Read the model definition and answer for the solid it produces. Units are mm, in the model's axes. A direction names the side the tool comes from. Coordinates: 2 decimals unless noted, no trailing zeros. Loops run counter-clockwise (first coordinate to the right, second up) from the corner with the lowest first, then second, coordinate; pieces in that order, holes last.
from build123d import *

# Parameters (mm, degrees)
SKETCH_1_R          = 1.45
EXTRUDE_1_DEPTH     = 5
EXTRUDE_2_DEPTH     = 5
FILLET_1_R          = 10
FILLET_2_R          = 2.5
CUT_EXTRUDE_1_DEPTH = 183.793945183
FILLET_3_R          = 3


with BuildPart() as part:
    # 草图1 → 凸台-拉伸1 (new body)
    with BuildSketch(Plane.XY):
        Polygon((-7.5, -7.5), (-7.5, 135.890872965), (13.765981284, 135.890872965), (23.715728753, 125.941125497), (5, 107.225396744), (5, 5), (39.953318806, 5), (79.577164466, 44.623845661), (73.213203436, 50.987806691), (85.941125497, 63.715728753), (122.156854249, 27.5), (122.156854249, -7.5), align=None)
        Circle(SKETCH_1_R, mode=Mode.SUBTRACT)
        with Locations((0, 15)):
            Circle(SKETCH_1_R, mode=Mode.SUBTRACT)
        with Locations((0, 35)):
            Circle(SKETCH_1_R, mode=Mode.SUBTRACT)
        with Locations((15, 0)):
            Circle(SKETCH_1_R, mode=Mode.SUBTRACT)
        with Locations((35, 0)):
            Circle(SKETCH_1_R, mode=Mode.SUBTRACT)
        with Locations((18.058874503, 125.941125497)):
            Circle(SKETCH_1_R, mode=Mode.SUBTRACT)
        with Locations((13.109127035, 130.890872965)):
            Circle(SKETCH_1_R, mode=Mode.SUBTRACT)
        with Locations((6.038059223, 123.819805153)):
            Circle(SKETCH_1_R, mode=Mode.SUBTRACT)
        with Locations((10.987806691, 118.870057685)):
            Circle(SKETCH_1_R, mode=Mode.SUBTRACT)
        with Locations((90.890872965, 53.109127035)):
            Circle(SKETCH_1_R, mode=Mode.SUBTRACT)
        with Locations((85.941125497, 58.058874503)):
            Circle(SKETCH_1_R, mode=Mode.SUBTRACT)
        with Locations((78.870057685, 50.987806691)):
            Circle(SKETCH_1_R, mode=Mode.SUBTRACT)
        with Locations((83.819805153, 46.038059223)):
            Circle(SKETCH_1_R, mode=Mode.SUBTRACT)
        with Locations((0, 125)):
            Circle(SKETCH_1_R, mode=Mode.SUBTRACT)
        with Locations((0, 105)):
            Circle(SKETCH_1_R, mode=Mode.SUBTRACT)
        with Locations((70, 0)):
            Circle(SKETCH_1_R, mode=Mode.SUBTRACT)
        with Locations((90, 0)):
            Circle(SKETCH_1_R, mode=Mode.SUBTRACT)
        Polygon((94.567828227, 48.01795821), (51.549870017, 5), (115.156854249, 5), (115.156854249, 27.428932188), align=None, mode=Mode.SUBTRACT)
    extrude(amount=EXTRUDE_1_DEPTH)

    # 草图3 → 凸台-拉伸2 (add)
    with BuildSketch(Plane.XY):
        Polygon((97.567828227, 45.01795821), (97.567828227, 5), (85.567828227, 5), (68.558849122, 22.008979105), (74.215703372, 27.665833355), (87.567828227, 14.313708499), (87.567828227, 41.01795821), (94.567828227, 48.01795821), align=None)
        Polygon((73.213203436, 50.987806691), (5, 29.379876147), (5, 21), (24.533181149, 27.187535555), (31.561537876, 5), (39.953318806, 5), (32.159691009, 29.603388895), (79.577164466, 44.623845661), align=None)
    extrude(amount=EXTRUDE_2_DEPTH)

    # 圆角1
    fillet_1_edges = [part.edges().sort_by_distance(p)[0] for p in [
        (5, 29.379876147, 2.5),
    ]]
    fillet(fillet_1_edges, radius=FILLET_1_R)

    # 圆角2
    fillet_2_edges = [part.edges().sort_by_distance(p)[0] for p in [
        (97.567828227, 5, 2.5),
        (85.567828227, 5, 2.5),
        (68.558849122, 22.008979105, 2.5),
        (74.215703372, 27.665833355, 2.5),
        (87.567828227, 14.313708499, 2.5),
        (87.567828227, 41.01795821, 2.5),
        (97.567828227, 45.01795821, 2.5),
        (32.159691009, 29.603388895, 2.5),
        (31.561537876, 5, 2.5),
        (24.533181149, 27.187535555, 2.5),
        (5, 21, 2.5),
        (5, 5, 2.5),
        (39.953318806, 5, 2.5),
        (79.577164466, 44.623845661, 2.5),
        (115.156854249, 27.428932188, 2.5),
        (51.549870017, 5, 2.5),
        (115.156854249, 5, 2.5),
    ]]
    fillet(fillet_2_edges, radius=FILLET_2_R)

    # 草图4 → 切除-拉伸1 (cut, through all)
    with BuildSketch(Plane.XY.offset(5)):
        Polygon((97.567828227, -7.5), (97.567828227, 52.089026022), (122.156854249, 27.5), (122.156854249, -7.5), align=None)
    extrude(amount=-CUT_EXTRUDE_1_DEPTH, mode=Mode.SUBTRACT)

    # 圆角3
    fillet_3_edges = [part.edges().sort_by_distance(p)[0] for p in [
        (-7.5, -7.5, 2.5),
        (-7.5, 135.890872965, 2.5),
        (13.765981284, 135.890872965, 2.5),
        (23.715728753, 125.941125497, 2.5),
        (5, 107.225396744, 2.5),
        (73.213203436, 50.987806691, 2.5),
        (85.941125497, 63.715728753, 2.5),
        (97.567828227, -7.5, 2.5),
        (97.567828227, 52.089026022, 2.5),
    ]]
    fillet(fillet_3_edges, radius=FILLET_3_R)


solid = part.part
Item 1: A cutting plane is placed at C-C on y = 15. Determine the outline of the cut face in (x, z).
Numbers:
outline: (-7.5, 0) - (-1.45, 0) - (-1.45, 5) - (-7.5, 5) - close; (1.45, 0) - (5, 0) - (5, 5) - (1.45, 5) - close; (28.39, 0) - (36.79, 0) - (36.79, 5) - (28.39, 5) - close; (49.95, 0) - (61.55, 0) - (61.55, 5) - (49.95, 5) - close; (75.57, 0) - (97.57, 0) - (97.57, 5) - (75.57, 5) - close
Item 2: Which of the six approach directions +Z, -Z, +X, -X, +Y, -Y give full straight-line access (tool end or side, diameter ignored) to faces 4 (the face through (96.67, -6.64, 2.46)), 5 (the face through (13.847, 116.072, 2.465)), 6 (the face through (8.987, 35.047, 2.535))?
Numbers:
face 4: +Z, -Z, +X, -Y
face 5: +Z, -Z, +X
face 6: +Z, -Z
Item 3: Given pin 1 (1 mm diameter, centred on y = 121, z = 4.5, fed in from +X); pin 2 (1.5 mm diameter, centred on x = 22.5, z = 2.5, fed in from +Y); pin 3 (1 mm diameter, centred on y = 59, z = 2.5, fed in from +X), each flat-ended and moving along its own axis, determine where each tip first touches the part or whether it passes through.
Numbers:
pin 1: stops at x = 19.27
pin 2: stops at y = 127.89
pin 3: stops at x = 91.16
Item 4: Determine the mould class of faces 1 (the face through (46, -7.5, 2)), 2 (the face through (-7.5, 63, 2)), 3 (the face through (35.853, 17.943, 2.465)) for opening direction Y: released by +Y, released by -Y, zero draft, split by the parting line, or undercut.
Numbers:
face 1: released by -Y
face 2: zero draft
face 3: undercut
Item 5: A cutting plane is placed at D-D on x = 49.5. Determine the outline of the cut face in (y, z).
Numbers:
outline: (-7.5, 0) - (14.55, 0) - (14.55, 5) - (-7.5, 5) - close; (35.1, 0) - (43.48, 0) - (43.48, 5) - (35.1, 5) - close
Item 6: Find the intervals of material crossed by line 1 along Y through (x, z) = (0, 1.9); line 2 along Y through (x, z) = (60, 3.9); line 3 along Y through (x, z) = (62, 0.6), in increasing order.
Numbers:
line 1: y = -7.5 to -1.45, 1.45 to 13.55, 16.45 to 33.55, 36.45 to 103.55, 106.45 to 123.55, 126.45 to 135.89
line 2: y = -7.5 to 5, 13.45 to 25.05, 38.42 to 46.8
line 3: y = -7.5 to 5, 15.45 to 27.05, 39.06 to 47.44
Item 7: A cutting plane is placed at B-B on x = 0. Determine the outline of the cut face in (y, z), then the cut area to 3 significant figures.
Numbers:
outline: (-7.5, 0) - (-1.45, 0) - (-1.45, 5) - (-7.5, 5) - close; (1.45, 0) - (13.55, 0) - (13.55, 5) - (1.45, 5) - close; (16.45, 0) - (33.55, 0) - (33.55, 5) - (16.45, 5) - close; (36.45, 0) - (103.55, 0) - (103.55, 5) - (36.45, 5) - close; (106.45, 0) - (123.55, 0) - (123.55, 5) - (106.45, 5) - close; (126.45, 0) - (135.89, 0) - (135.89, 5) - (126.45, 5) - close
area: 644 mm2
Item 8: A cutting plane is placed at A-A on y = 0. Determine the outline of the cut face in (x, z).
Numbers:
outline: (-7.5, 0) - (-1.45, 0) - (-1.45, 5) - (-7.5, 5) - close; (1.45, 0) - (13.55, 0) - (13.55, 5) - (1.45, 5) - close; (16.45, 0) - (33.55, 0) - (33.55, 5) - (16.45, 5) - close; (36.45, 0) - (68.55, 0) - (68.55, 5) - (36.45, 5) - close; (71.45, 0) - (88.55, 0) - (88.55, 5) - (71.45, 5) - close; (91.45, 0) - (97.57, 0) - (97.57, 5) - (91.45, 5) - close
